from build123d import *

# Parameters (mm, degrees)
SKETCH3_W           = 70
SKETCH3_H           = 800
SKETCH3_W_2         = 2500
SKETCH3_H_2         = 70
BOSS_EXTRUDE1_DEPTH = 40
SKETCH4_W           = 70
SKETCH4_H           = 40
BOSS_EXTRUDE2_DEPTH = 300
SKETCH5_R           = 10
CUT_EXTRUDE1_DEPTH  = 10
SKETCH6_R           = 20
CUT_EXTRUDE2_DEPTH  = 1634.806904135
SKETCH7_R           = 7.5
CUT_EXTRUDE3_DEPTH  = 20
SKETCH8_W           = 70
SKETCH8_H           = 80
BOSS_EXTRUDE3_DEPTH = 80
SKETCH10_R          = 12.5
CUT_EXTRUDE4_DEPTH  = 60
SKETCH11_W          = 240
SKETCH11_H          = 180
SKETCH11_R          = 20
BOSS_EXTRUDE4_DEPTH = 40
SKETCH12_W          = 33
SKETCH12_H          = 180
CUT_EXTRUDE5_DEPTH  = 1722.866719581


with BuildPart() as part:
    # Sketch3 → Boss-Extrude1 (new body)
    with BuildSketch(Plane(origin=(300, 0, 0), x_dir=(0, 0, -1), z_dir=(1, 0, 0))):
        with Locations((105, -435)):
            Rectangle(SKETCH3_W, SKETCH3_H)
        Rectangle(SKETCH3_W_2, SKETCH3_H_2)
        with Locations((-915, -435)):
            Rectangle(SKETCH3_W, SKETCH3_H)
        with Locations((1015, -435)):
            Rectangle(SKETCH3_W, SKETCH3_H)
    boss_extrude1 = extrude(amount=BOSS_EXTRUDE1_DEPTH)

    # Sketch4 → Boss-Extrude2 (add)
    with BuildSketch(Plane.ZY.offset(-300)):
        with Locations((-1015, -205)):
            Rectangle(SKETCH4_W, SKETCH4_H)
        with Locations((-105, -205)):
            Rectangle(SKETCH4_W, SKETCH4_H)
        with Locations((915, -205)):
            Rectangle(SKETCH4_W, SKETCH4_H)
        with Locations((-1015, -695)):
            Rectangle(SKETCH4_W, SKETCH4_H)
        with Locations((-105, -695)):
            Rectangle(SKETCH4_W, SKETCH4_H)
        with Locations((915, -695)):
            Rectangle(SKETCH4_W, SKETCH4_H)
    boss_extrude2 = extrude(amount=BOSS_EXTRUDE2_DEPTH)

    # Mirror2: Boss-Extrude2 across plane
    add(boss_extrude2.mirror(Plane(origin=(0, 0, 0), x_dir=(0, 0, 1), z_dir=(1, 0, 0))))

    # Mirror3: Boss-Extrude1 across plane
    add(boss_extrude1.mirror(Plane(origin=(0, 0, 0), x_dir=(0, 0, 1), z_dir=(1, 0, 0))))

    # Sketch5 → Cut-Extrude1 (cut)
    with BuildSketch(Plane(origin=(-300, 0, 0), x_dir=(0, 0, -1), z_dir=(1, 0, 0))):
        with Locations((-1050, 12.5)):
            Circle(SKETCH5_R)
        with Locations((-980, 12.5)):
            Circle(SKETCH5_R)
        with Locations((-910, 12.5)):
            Circle(SKETCH5_R)
        with Locations((-840, 12.5)):
            Circle(SKETCH5_R)
        with Locations((-770, 12.5)):
            Circle(SKETCH5_R)
        with Locations((-700, 12.5)):
            Circle(SKETCH5_R)
        with Locations((-630, 12.5)):
            Circle(SKETCH5_R)
        with Locations((-560, 12.5)):
            Circle(SKETCH5_R)
        with Locations((-490, 12.5)):
            Circle(SKETCH5_R)
        with Locations((-420, 12.5)):
            Circle(SKETCH5_R)
        with Locations((-350, 12.5)):
            Circle(SKETCH5_R)
        with Locations((-280, 12.5)):
            Circle(SKETCH5_R)
        with Locations((-210, 12.5)):
            Circle(SKETCH5_R)
        with Locations((-140, 12.5)):
            Circle(SKETCH5_R)
        with Locations((-70, 12.5)):
            Circle(SKETCH5_R)
        with Locations((0, 12.5)):
            Circle(SKETCH5_R)
        with Locations((70, 12.5)):
            Circle(SKETCH5_R)
        with Locations((140, 12.5)):
            Circle(SKETCH5_R)
        with Locations((210, 12.5)):
            Circle(SKETCH5_R)
        with Locations((280, 12.5)):
            Circle(SKETCH5_R)
        with Locations((350, 12.5)):
            Circle(SKETCH5_R)
        with Locations((420, 12.5)):
            Circle(SKETCH5_R)
        with Locations((490, 12.5)):
            Circle(SKETCH5_R)
        with Locations((560, 12.5)):
            Circle(SKETCH5_R)
        with Locations((630, 12.5)):
            Circle(SKETCH5_R)
        with Locations((700, 12.5)):
            Circle(SKETCH5_R)
        with Locations((770, 12.5)):
            Circle(SKETCH5_R)
        with Locations((840, 12.5)):
            Circle(SKETCH5_R)
        with Locations((910, 12.5)):
            Circle(SKETCH5_R)
        with Locations((980, 12.5)):
            Circle(SKETCH5_R)
        with Locations((1050, 12.5)):
            Circle(SKETCH5_R)
    cut_extrude1 = extrude(amount=-CUT_EXTRUDE1_DEPTH, mode=Mode.SUBTRACT)

    # Mirror4: Cut-Extrude1 across plane
    add(cut_extrude1.mirror(Plane(origin=(0, 0, 0), x_dir=(0, 0, 1), z_dir=(1, 0, 0))), mode=Mode.SUBTRACT)

    # Sketch6 → Cut-Extrude2 (cut, symmetric)
    with BuildSketch(Plane(origin=(-300, 0, 0), x_dir=(0, 0, -1), z_dir=(1, 0, 0))):
        with Locations((-1180, 0)):
            Circle(SKETCH6_R)
    cut_extrude2 = extrude(amount=CUT_EXTRUDE2_DEPTH, both=True, mode=Mode.SUBTRACT)

    # Sketch7 → Cut-Extrude3 (cut)
    with BuildSketch(Plane.XZ.offset(835)):
        with Locations(Location((-320, 915, 0), (0, 0, 270))):
            Circle(SKETCH7_R)
        with Locations(Location((320, 915, 0), (0, 0, 270))):
            Circle(SKETCH7_R)
        with Locations(Location((320, -105, 0), (0, 0, 270))):
            Circle(SKETCH7_R)
        with Locations(Location((-320, -105, 0), (0, 0, 270))):
            Circle(SKETCH7_R)
        with Locations(Location((320, -1015, 0), (0, 0, 270))):
            Circle(SKETCH7_R)
        with Locations(Location((-320, -1015, 0), (0, 0, 270))):
            Circle(SKETCH7_R)
    extrude(amount=-CUT_EXTRUDE3_DEPTH, mode=Mode.SUBTRACT)

    # Mirror5: Cut-Extrude2 across plane
    add(cut_extrude2.mirror(Plane.XY), mode=Mode.SUBTRACT)

    # Sketch8 → Boss-Extrude3 (add)
    with BuildSketch(Plane.ZY.offset(340)):
        with Locations((-325, 5)):
            Rectangle(SKETCH8_W, SKETCH8_H)
        with Locations((445, 5)):
            Rectangle(SKETCH8_W, SKETCH8_H)
        with Locations((-1095, 5)):
            Rectangle(SKETCH8_W, SKETCH8_H)
    extrude(amount=BOSS_EXTRUDE3_DEPTH)

    # Sketch10 → Cut-Extrude4 (cut)
    with BuildSketch(Plane(origin=(0, 45, 0), x_dir=(1, 0, 0), z_dir=(0, 1, 0))):
        with Locations(Location((-382.500751055, 1095, 0), (0, 0, 270))):
            Circle(SKETCH10_R)
        with Locations(Location((-382.500751055, 325, 0), (0, 0, 270))):
            Circle(SKETCH10_R)
        with Locations(Location((-382.500751055, -445, 0), (0, 0, 270))):
            Circle(SKETCH10_R)
    extrude(amount=-CUT_EXTRUDE4_DEPTH, mode=Mode.SUBTRACT)

    # Sketch11 → Boss-Extrude4 (add)
    with BuildSketch(Plane(origin=(340, 0, 0), x_dir=(0, 0, -1), z_dir=(1, 0, 0))):
        with Locations((-1180, 0)):
            Rectangle(SKETCH11_W, SKETCH11_H)
        with Locations((-1180, 0)):
            Circle(SKETCH11_R, mode=Mode.SUBTRACT)
    extrude(amount=-BOSS_EXTRUDE4_DEPTH)

    # Sketch12 → Cut-Extrude5 (cut, through all)
    with BuildSketch(Plane(origin=(340, 0, 0), x_dir=(0, 0, -1), z_dir=(1, 0, 0))):
        with Locations((-1283.5, 0)):
            Rectangle(SKETCH12_W, SKETCH12_H)
    extrude(amount=-CUT_EXTRUDE5_DEPTH, mode=Mode.SUBTRACT)


solid = part.part
Can you work these out from the model? Positions are in its coordinate system, mm. A direction names the side the tool comes from. Give positions to 0.01 mm unless a question says otherwise; leave off trailing zeros. Loops run counter-clockwise (first coordinate to the right, second up) from the corner with the lowest first, then second, coordinate; pieces in that order, holes last. Notation, with made-up numbers: (23, 56.25) - (82, 56.25) arc R18 cw to (82, 66.25) - close; hole circle Ø11 at (29.5, 51.5). An arc over 180 degrees is marked (long way). Answer as a JSON object with one key per item and string values.
Q1. If we mould it in two halves opening along X, with no side actions, what happens to faces 1 (the flat face through (300, -447, -1015)), 2 (the flat face through (-49, -200, 950)), 3 (the flat face through (-420, 6, -325))? For each: pulls with the +X half, pulls with the -X half, needs draft (parallel to the pull), parting line crosses it, or undercut.
Geometry says:
{"face 1": "undercut", "face 2": "needs draft", "face 3": "pulls with the -X half"}
Q2. Which directions (+Z, -Z, +X, -X, +Y, -Y) give clear straight access to the entire face, cutting with the end or side of a thin tool? Please do faces 4 (the flat face through (300, -774, 915)), 5 (the flat face through (4, -675, -1015)), 6 (the flat face through (-49, -200, -980)), 7 (the flat face through (-340, 0, -1202)), 8 (the flat face through (-4, -185, -1015)).
Geometry says:
{"face 4": "+Z, -Z, -Y", "face 5": "+Z, -Z", "face 6": "+X, -X, -Y", "face 7": "-Z, -X, +Y, -Y", "face 8": "+Z, -Z, +Y"}
Q3. Will these pins go through, and if not, where does the flat tip stop? P1, Ø5, axis at y = 38.5, z = -312.5, coming from the +X side; P2, Ø16, axis at y = 12.5, z = 770, coming from the -X side; P3, Ø12, axis at x = 320, z = -105, coming from the -Y side.
Geometry says:
{"P1": "x = -340", "P2": "x = -340", "P3": "y = -815"}
Q4. Imagine slicing it at B-B on y = -365.5. Write out the boundary of the cut face in (x, z).
Geometry says:
{"outline": "(-340, -1050) - (-300, -1050) - (-300, -980) - (-340, -980) - close; (-340, -140) - (-300, -140) - (-300, -70) - (-340, -70) - close; (-340, 880) - (-300, 880) - (-300, 950) - (-340, 950) - close; (300, -1050) - (340, -1050) - (340, -980) - (300, -980) - close; (300, -140) - (340, -140) - (340, -70) - (300, -70) - close; (300, 880) - (340, 880) - (340, 950) - (300, 950) - close"}
Q5. Imagine slicing it at A-A on x = 50. Write out the boundary of the cut face in (y, z).
Geometry says:
{"outline": "(-715, -1050) - (-675, -1050) - (-675, -980) - (-715, -980) - close; (-715, -140) - (-675, -140) - (-675, -70) - (-715, -70) - close; (-715, 880) - (-675, 880) - (-675, 950) - (-715, 950) - close; (-225, -1050) - (-185, -1050) - (-185, -980) - (-225, -980) - close; (-225, -140) - (-185, -140) - (-185, -70) - (-225, -70) - close; (-225, 880) - (-185, 880) - (-185, 950) - (-225, 950) - close"}
Q6. If I drill on L1, parallel to X at y = -829.25, z = -105; L2, parallel to X at y = -730, z = -85; L3, parallel to Z at x = -305, y = -724.5, over which ranges is the centre line in solid material (lowest first)?
Geometry says:
{"L1": "-340 to -327.5, -312.5 to -300, 300 to 312.5, 327.5 to 340", "L2": "-340 to -300, 300 to 340", "L3": "-1050 to -980, -140 to -70, 880 to 950"}
